The listing builds one solid part. Answer for the finished solid, in the listing's coordinates (mm). Face numbers are marked on the shaded views. Give positions to 0.01 mm unless a question says otherwise; leave off trailing zeros. Write each loop counter-clockwise with the first axis right and the second up, starting at its lowest first coordinate (ties: lowest second). Pieces come first, ordered by that corner, then holes. Notation, with made-up numbers: (32, -4) - (39, -4) arc R19 cw to (39, 4) - close; hole circle Ø8 at (30, 78). An arc over 180 degrees is marked (long way). Write each question's results on one line, items separated by ' | '. Start each with the question number.
Q1. Flat-ended cylindrical pins translate along their axes: pin 1 Ø8 at (x, y) = (0, 0) entering from +Z; pin 2 Ø6.5 at (x, y) = (0, 0) entering from -Z. Find the tip coordinate at first contact, or state that the pin passes through.
Q2. Find the intervals of material crossed by probe 1 along X at (y, z) = (0, 0.75); probe 2 along X at (y, z) = (2, 0.9); probe 3 along Y at (x, z) = (0, -1), in increasing order.
Q3. For a pull along X with two mould halves and no side action, classify the marked faces 1, 2, 3 and 4 as pulls with the +X half, pulls with the -X half, needs draft (parallel to the pull), parting line crosses it, or undercut.
Q4. Section C-C (z = -0.35) is taken. Determine the outline of the cut face in (x, y), plus the area to 3 significant figures.
Q5. Section A-A (y = 0) is taken. Determine the outline of the cut face in (x, z).
Q6. Section D-D (x = -3) is taken. Determine the outline of the cut face in (y, z), plus the area to 3 significant figures.
```python
from build123d import *

# Parameters (mm, degrees)
SKETCH1_R           = 2.5
BOSS_EXTRUDE1_DEPTH = 1.5
SKETCH2_R           = 5
CUT_EXTRUDE1_DEPTH  = 1.5


with BuildPart() as part:
    # Sketch1 → Boss-Extrude1 (new body, symmetric)
    with BuildSketch(Plane.XY):
        with BuildLine():
            Line((-8.5, 10), (8.5, 10))
            ThreePointArc((8.5, 10), (9.560660172, 9.560660172), (10, 8.5))
            Line((10, 8.5), (10, -8.5))
            ThreePointArc((10, -8.5), (9.560660172, -9.560660172), (8.5, -10))
            Line((8.5, -10), (-8.5, -10))
            ThreePointArc((-8.5, -10), (-9.560660172, -9.560660172), (-10, -8.5))
            Line((-10, -8.5), (-10, 8.5))
            ThreePointArc((-10, 8.5), (-9.560660172, 9.560660172), (-8.5, 10))
        make_face()
        Circle(SKETCH1_R, mode=Mode.SUBTRACT)
    extrude(amount=BOSS_EXTRUDE1_DEPTH, both=True)

    # Sketch2 → Cut-Extrude1 (cut)
    with BuildSketch(Plane(origin=(0, 0, -1.5), x_dir=(-1, 0, 0), z_dir=(0, 0, -1))):
        Circle(SKETCH2_R)
    extrude(amount=-CUT_EXTRUDE1_DEPTH, mode=Mode.SUBTRACT)


solid = part.part
```
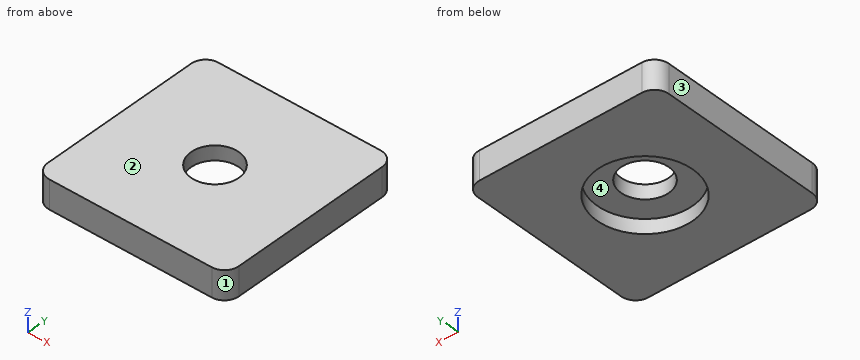
Answers below:
1) pin 1: stops at z = 1.5 | pin 2: stops at z = 0
2) probe 1: x = -10 to -2.5, 2.5 to 10 | probe 2: x = -10 to -1.5, 1.5 to 10 | probe 3: y = -10 to -5, 5 to 10
3) face 1: pulls with the +X half | face 2: needs draft | face 3: pulls with the -X half | face 4: undercut
4) outline: (-10, -8.5) arc R1.5 ccw to (-8.5, -10) - (8.5, -10) arc R1.5 ccw to (10, -8.5) - (10, 8.5) arc R1.5 ccw to (8.5, 10) - (-8.5, 10) arc R1.5 ccw to (-10, 8.5) - close; hole circle Ø10 at (0, 0) | area: 320 mm2
5) outline: (-10, -1.5) - (-5, -1.5) - (-5, 0) - (-2.5, 0) - (-2.5, 1.5) - (-10, 1.5) - close; (2.5, 0) - (5, 0) - (5, -1.5) - (10, -1.5) - (10, 1.5) - (2.5, 1.5) - close
6) outline: (-10, -1.5) - (-4, -1.5) - (-4, 0) - (4, 0) - (4, -1.5) - (10, -1.5) - (10, 1.5) - (-10, 1.5) - close | area: 48.0 mm2
